Job drawing, mm, ordinate dimensions from the low corner. One solid piece. A direction names the side the tool comes from. Coordinates: 2 decimals unless noted, no trailing zeros. Write each loop counter-clockwise with the first axis right and the second up, starting at its lowest first coordinate (ties: lowest second). Pieces come first, ordered by that corner, then holes.
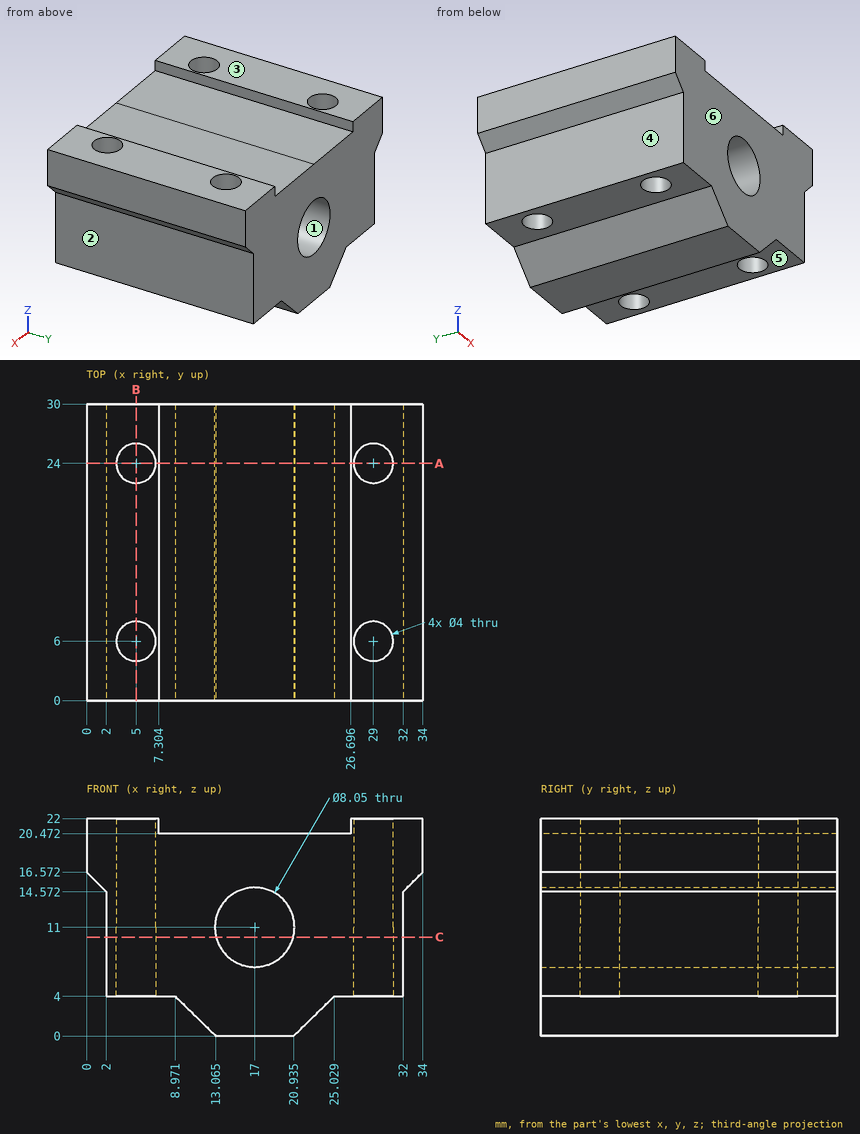
1. Saw through at C-C on z = 10. List the corners of the cut face in (x, y).
Computed values:
outline: (2, 0) - (13.1, 0) - (13.1, 30) - (2, 30) - close; (20.9, 0) - (32, 0) - (32, 30) - (20.9, 30) - close; hole circle Ø4 at (5, 6); hole circle Ø4 at (5, 24); hole circle Ø4 at (29, 6); hole circle Ø4 at (29, 24)
2. Saw through at A-A on y = 24. State how many separate pieces and enclosed holes the cut face has, plus the area to 3 significant figures.
Computed values:
separate pieces: 3
enclosed holes: 1
area: 389 mm2
3. 3-axis set-ups, long thin cutter, end or side, ignore diameter. For the marked faces 4, 5 and 6: which of +Z, -Z, +X, -X, +Y, -Y reach the whole face in a straight line?
Computed values:
face 4: -Z, -X, +Y, -Y
face 5: -Z, +X, +Y, -Y
face 6: +Z, -Z, +X, -X, -Y
4. Mould opens along X. For the marked faces 1, 2 and 3 say: +X half, -X half, draft (parallel to the pull), parting line (faces both ways), or undercut.
Computed values:
face 1: undercut
face 2: +X half
face 3: draft
5. Saw through at B-B on x = 5. List the corners of the cut face in (y, z).
Computed values:
outline: (0, 4) - (4, 4) - (4, 22) - (0, 22) - close; (8, 4) - (22, 4) - (22, 22) - (8, 22) - close; (26, 4) - (30, 4) - (30, 22) - (26, 22) - close
6. Probe line 1 along Y through (x, z) = (5, 18.5); line 2 along X through (y, z) = (25.25, 6.75); line 3 along X through (y, z) = (6.75, 18.25) (1 decimal). List the from-to ranges inside material, lowest first.
Computed values:
line 1: y = 0 to 4, 8 to 22, 26 to 30
line 2: x = 2 to 3.44, 6.56 to 27.44, 30.56 to 32
line 3: x = 0 to 3.1, 6.9 to 27.1, 30.9 to 34
7. Flat gauge pins, fed straight in: pin 1 (3 mm diameter, centred on x = 10, y = 15, fed in from +Z); pin 2 (3.5 mm diameter, centred on x = 30, y = 21.5, fed in from -Z); pin 3 (2.5 mm diameter, centred on x = 5, y = 24, fed in from -Z); pin 4 (1 mm diameter, centred on y = 15.5, z = 6.5, fed in from -X). Where does each tip first touch, or does it go through?
Computed values:
pin 1: stops at z = 20.47
pin 2: stops at z = 4
pin 3: passes through
pin 4: stops at x = 2
